```python
from build123d import *

# Parameters (mm, degrees)
F0_W      = 90
F0_H      = 70
F0_R      = 1.5
F2_DEPTH  = 5
F4_D      = 3
F5_D      = 11.5
F7_DEPTH  = 5
F9_DEPTH  = 0.1
F10_R     = 11
F10_R_2   = 5.75
F11_DEPTH = 5.001
F13_DEPTH = 5.001


with BuildPart() as f2:
    # F0 (on Top) → F2 (new body)
    with BuildSketch(Plane.XY):
        Rectangle(F0_W, F0_H)
        with Locations((-9, -28.5)):
            Circle(F0_R, mode=Mode.SUBTRACT)
        with Locations((36, -20)):
            Circle(F0_R, mode=Mode.SUBTRACT)
        with Locations((-9, 28.5)):
            Circle(F0_R, mode=Mode.SUBTRACT)
        with Locations((36, 20)):
            Circle(F0_R, mode=Mode.SUBTRACT)
    extrude(amount=F2_DEPTH)

    # F4 (through all)
    with Locations(Plane.XY.offset(5)):
        with Locations((-2.420886, 15.522152), (-2.420886, -15.379748), (-33.465192, -15.379748), (-33.465192, 15.522152)):
            Hole(F4_D / 2)

    # F5 (through all)
    with Locations(Plane(origin=(0, 0, 0), x_dir=(1, 0, 0), z_dir=(0, 0, -1))):
        with Locations((-18, 0)):
            Hole(F5_D / 2)

    # F6 (on face) → F7 (cut)
    with BuildSketch(Plane.XY.offset(5)):
        Polygon((7.15526, 35), (45, 24.844227), (45, 35), align=None)
    extrude(amount=-F7_DEPTH, mode=Mode.SUBTRACT)

    # F8 (on face) → F9 (cut)
    with BuildSketch(Plane.XY.offset(5)):
        Polygon((45, -25.128944), (7.019877, -35), (45, -35), align=None)
    extrude(amount=F9_DEPTH, mode=Mode.SUBTRACT)

    # F10 (on face) → F11 (cut, through all)
    with BuildSketch(Plane.XY.offset(5)):
        with Locations((-18, 0)):
            Circle(F10_R)
        with Locations((-18, 0)):
            Circle(F10_R_2, mode=Mode.SUBTRACT)
    extrude(amount=-F11_DEPTH, mode=Mode.SUBTRACT)

    # F12 (on face) → F13 (cut, through all)
    with BuildSketch(Plane.XY.offset(5)):
        Polygon((45, -24.844), (7.15526, -35), (45, -35), align=None)
    extrude(amount=-F13_DEPTH, mode=Mode.SUBTRACT)


solid = f2.part
```
Geometry: final body of the model. Coordinates: model frame, mm. Give positions to 0.01 mm unless a question says otherwise; leave off trailing zeros. Write each loop counter-clockwise with the first axis right and the second up, starting at its lowest first coordinate (ties: lowest second). Pieces come first, ordered by that corner, then holes.
1. Draft query along Y for faces 1 (the flat face through (-19, 35, 2)), 2 (the flat face through (-45, 0, 2)), 3 (the cylindrical face through (34.89, 21.01, 2.46)). Return one class per face: released by +Y, released by -Y, zero draft, split by the parting line, or undercut.
2. Section query C-C, the plane x = -9. Return loops of the section in (y, z), then the cut area to 3 significant figures.
3. Pin query (flat end, axial travel): P1, Ø1.5, axis at x = -13.5, y = -21.5, coming from the -Z side. Return the tip coordinate at first contact, or that it passes through.
4. Line query: probe 1 along X at (y, z) = (-16, 2); probe 2 along Y at (x, z) = (35.5, 4.8); probe 3 along X at (y, z) = (-16.5, 3.85). Output: solid intervals per line, ascending.
5. Section query B-B, the plane x = -18. Return loops of the section in (y, z).
6. Section query D-D, the plane z = 3.6. Count the separate pieces of the cut face and the enclosed holes in it, then the cut area to 3 significant figures.
7. Section query A-A, the plane y = 20. Return loops of the section in (x, z), then the cut area to 3 significant figures.
Computed:
1. face 1: released by +Y
1. face 2: zero draft
1. face 3: undercut
2. outline: (-35, 0) - (-30, 0) - (-30, 5) - (-35, 5) - close; (-27, 0) - (-6.32, 0) - (-6.32, 5) - (-27, 5) - close; (6.32, 0) - (27, 0) - (27, 5) - (6.32, 5) - close; (30, 0) - (35, 0) - (35, 5) - (30, 5) - close
2. area: 257 mm2
3. P1: stops at z = 0
4. probe 1: x = -45 to -34.83, -32.1 to -3.79, -1.06 to 45
4. probe 2: y = -27.39 to -21.41, -18.59 to 18.59, 21.41 to 27.39
4. probe 3: x = -45 to -34.46, -32.47 to -3.42, -1.42 to 45
5. outline: (-35, 0) - (-11, 0) - (-11, 5) - (-35, 5) - close; (11, 0) - (35, 0) - (35, 5) - (11, 5) - close
6. separate pieces: 1
6. enclosed holes: 9
6. area: 5,480 mm2
7. outline: (-45, 0) - (34.5, 0) - (34.5, 5) - (-45, 5) - close; (37.5, 0) - (45, 0) - (45, 5) - (37.5, 5) - close
7. area: 435 mm2
